Print and shaded views of the part. All mm, measured from the part's lowest x, y and z. A direction names the side the tool comes from. Give positions to 0.01 mm unless a question says otherwise; leave off trailing zeros. Write each loop counter-clockwise with the first axis right and the second up, starting at its lowest first coordinate (ties: lowest second). Pieces come first, ordered by that corner, then holes. Notation, with made-up numbers: (15.25, -19.5) -> (41.25, -19.5) arc R8 ccw to (41.25, -15.5) -> close; hole circle Ø7 at (45.25, -4.5). An arc over 180 degrees is marked (long way). Put each result on its own line as item: value.
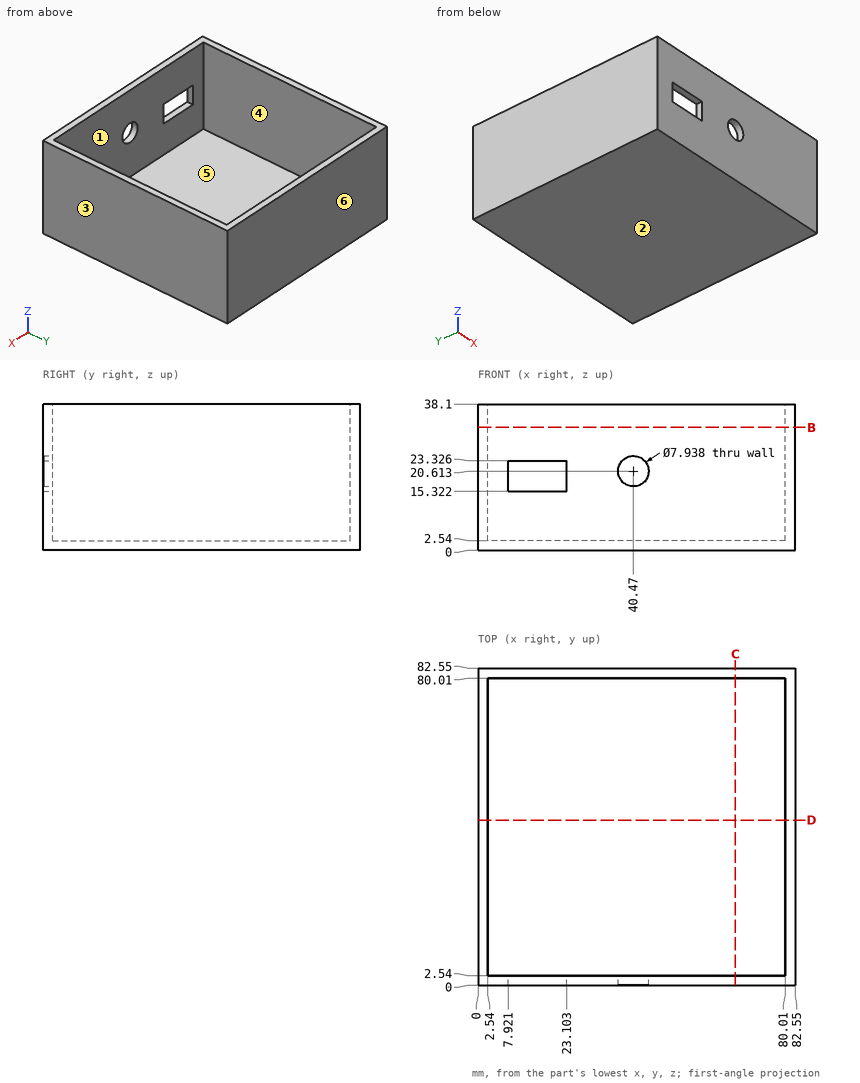
1) Slice it at C-C (x = 67). Write the cut outline in (y, z).
Filled sheet:
outline: (0, 0) -> (82.55, 0) -> (82.55, 38.1) -> (80.01, 38.1) -> (80.01, 2.54) -> (2.54, 2.54) -> (2.54, 38.1) -> (0, 38.1) -> close
2) Pull direction X, two halves, no side cores. Call the marked faces 1, 2, 3 and 4: released by +X, released by -X, zero draft, split by the parting line, or undercut.
Filled sheet:
face 1: undercut
face 2: zero draft
face 3: released by +X
face 4: undercut
3) Wall check: L1, parallel to Y at x = 24, z = 34; L2, parallel to Z at x = 62, y = 76.5. Give the ranges that are in metal, low to high.
Filled sheet:
L1: 0 to 2.54, 80.01 to 82.55
L2: 0 to 2.54
4) Tool access for the marked faces 5 and 6: list every direction of +Z, -Z, +X, -X, +Y, -Y with a clear straight run to the whole face (end or side of a thin tool).
Filled sheet:
face 5: +Z
face 6: +Z, -Z, +X, -X, +Y
5) Pin check, flat tip, straight feed: pin 1 (6 mm diameter, centred on x = 51.5, y = 27, fed in from +Z). Stop position of the tip, or through.
Filled sheet:
pin 1: z = 2.54
6) Slice it at B-B (z = 32). Write the cut outline in (x, y).
Filled sheet:
outline: (0, 0) -> (82.55, 0) -> (82.55, 82.55) -> (0, 82.55) -> close; hole (2.54, 2.54) -> (80.01, 2.54) -> (80.01, 80.01) -> (2.54, 80.01) -> close
